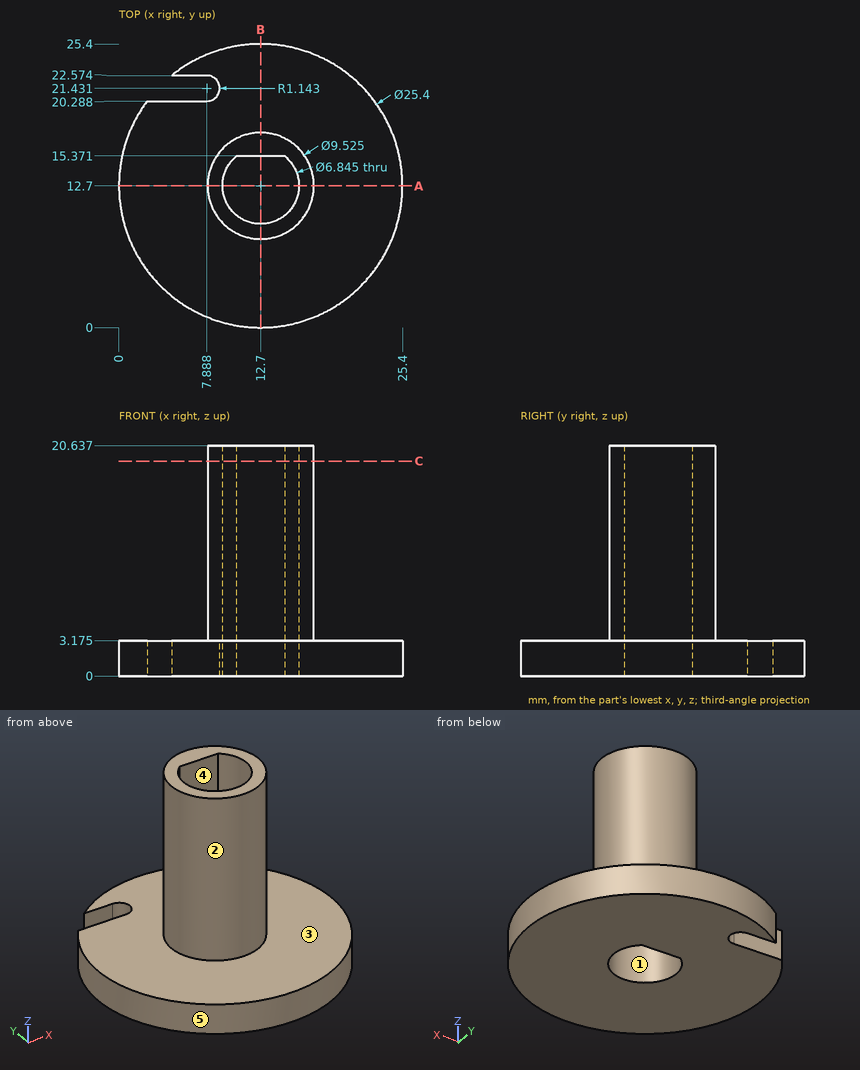
For this review, use the dimensioned drawing (mm, ordinates from the lowest corner) and the shaded views. A direction names the side the tool comes from. Coordinates: 2 decimals unless noted, no trailing zeros. Loops run counter-clockwise (first coordinate to the right, second up) from the corner with the lowest first, then second, coordinate; pieces in that order, holes last.
1. Mouldability with a two-part tool opening along X and no side actions: class the marked faces 3, 4 and 5 as +X half, -X half, draft (parallel to the pull), parting line (faces both ways), or undercut.
2. Add section A-A, the plane y = 12.7. Give the boundary of the cut face in (x, z) (1 decimal).
3. For the marked faces 1 and 2, list the 3-axis set-ups (+Z, -Z, +X, -X, +Y, -Y) from which the entire face can be reached by the end or side of a thin tool; tool diameter is ignored.
4. Add section B-B, the plane x = 12.7. Give the boundary of the cut face in (y, z) (1 decimal), then the cut area to 3 significant figures.
5. Insertion check: P1, Ø8, axis at y = 5.5, z = 7.5, coming from the +X side; P2, Ø2, axis at x = 21.5, y = 4.5, coming from the +Z side (1 decimal); P3, Ø6, axis at x = 10, z = 18.5, coming from the +Y side. Each pin has a flat end and moves straight along its axis. Give the tip position at first contact, or say it passes through.
6. Add section C-C, the plane z = 19.25. Give the boundary of the cut face in (x, y) (1 decimal).
7. For line 1 (Y direction, x = 12.7, z = 8.5); line 2 (Z direction, x = 20.75, y = 6.25) (1 decimal); line 3 (X direction, y = 13.25, z = 5.75), list the stretches that pass through material, from the lowest coordinate up.
Result:
1. face 3: draft
1. face 4: undercut
1. face 5: parting line
2. outline: (0, 0) - (9.3, 0) - (9.3, 20.6) - (7.9, 20.6) - (7.9, 3.2) - (0, 3.2) - close; (16.1, 0) - (25.4, 0) - (25.4, 3.2) - (17.5, 3.2) - (17.5, 20.6) - (16.1, 20.6) - close
3. face 1: +Z, -Z
3. face 2: +Z
4. outline: (0, 0) - (9.3, 0) - (9.3, 20.6) - (7.9, 20.6) - (7.9, 3.2) - (0, 3.2) - close; (15.4, 0) - (25.4, 0) - (25.4, 3.2) - (17.5, 3.2) - (17.5, 20.6) - (15.4, 20.6) - close
4. area: 121 mm2
5. P1: stops at x = 16.23
5. P2: stops at z = 3.2
5. P3: stops at y = 17.46
6. outline: circle Ø9.5 at (12.7, 12.7); hole (10.6, 15.4) arc R3.4 ccw (long way) to (14.8, 15.4) - close
7. line 1: y = 7.94 to 9.28, 15.37 to 17.46
7. line 2: z = 0 to 3.2
7. line 3: x = 7.97 to 9.32, 16.08 to 17.43
